Print and shaded views of the part. All mm, measured from the part's lowest x, y and z. A direction names the side the tool comes from. Coordinates: 2 decimals unless noted, no trailing zeros. Order: outer loops, then holes, each group sorted by start corner. A loop starts at its lowest first (then second) coordinate and runs counter-clockwise, first axis right, second up. Notation, with made-up numbers: (-26.75, -39.5) -> (28.25, -39.5) arc R25 cw to (28.25, -18.5) -> close; hole circle Ø10 at (73, -28.5). An arc over 180 degrees is marked (long way). Write item = value, one per line. Start each with the question number.
Q1. Cut at D-D, the plane y = 13.5. List the corners of the cut face in (x, z), plus the area to 3 significant figures.
Q2. 3-axis set-ups, long thin cutter, end or side, ignore diameter. For the marked faces 4, 5, 6, 7 and 8: which of +Z, -Z, +X, -X, +Y, -Y reach the whole face in a straight line?
Q3. Flat gauge pins, fed straight in: pin 1 (6.5 mm diameter, centred on x = 12.5, y = 5.5, fed in from -Z); pin 2 (4 mm diameter, centred on x = 14.5, z = 17.5, fed in from +Y); pin 3 (2 mm diameter, centred on x = 25.5, z = 36, fed in from -Y); pin 4 (4 mm diameter, centred on y = 12.5, z = 28, fed in from -X). Where does each tip first touch, or does it go through?
Q4. Cut at C-C, the plane z = 38. List the corners of the cut face in (x, y) (3 decimals).
Q5. Cut at A-A, the plane y = 24. List the corners of the cut face in (x, z).
Q6. Mould opens along X. For the marked faces 1, 2 and 3 say: +X half, -X half, draft (parallel to the pull), parting line (faces both ways), or undercut.
Q7. Cut at B-B, the plane x = 44. List the corners of the cut face in (y, z).
Q8. Wall check: line 1 (X direction, y = 31.5, z = 35.5); line 2 (Z direction, x = 28, y = 36.5); line 3 (Z direction, x = 61.5, y = 14). Give the ranges that are in metal, low to high. Write a range as from..to.
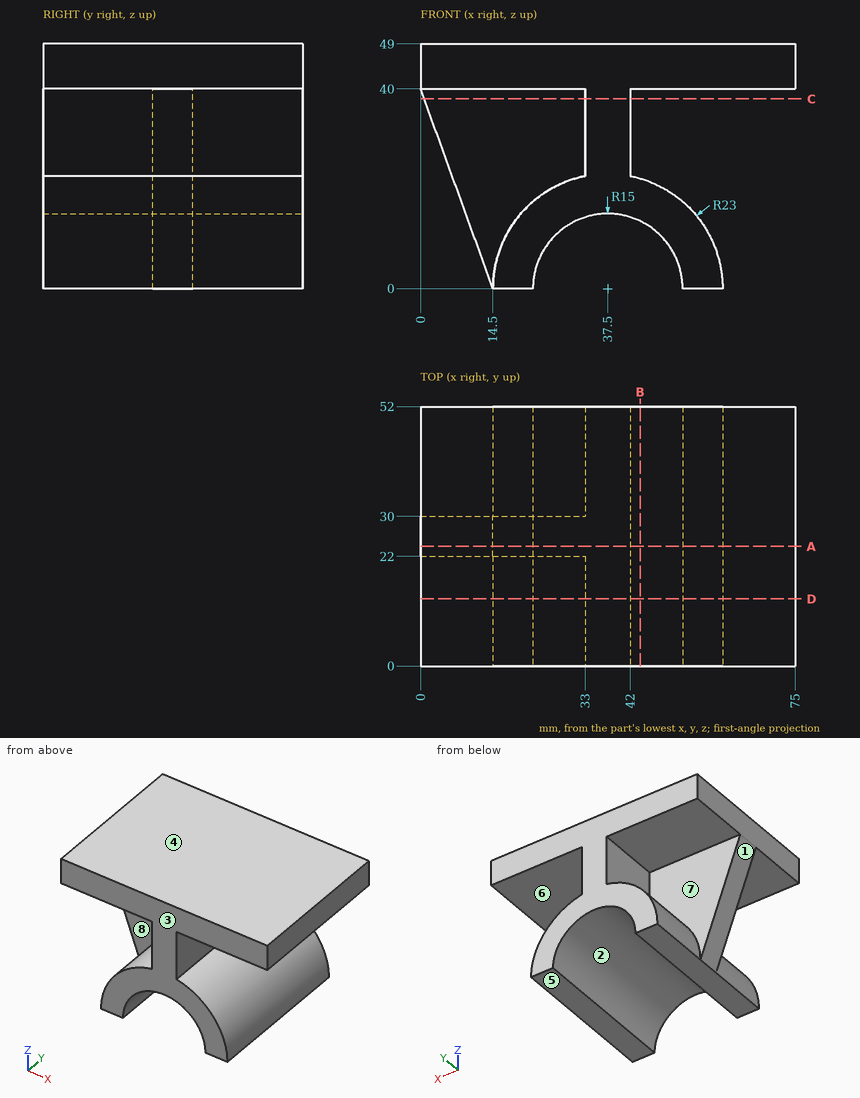
Here are the results:
q1.outline = (0, 40) -> (33, 40) -> (33, 22.56) arc R23 ccw to (14.5, 0) -> (22.5, 0) arc R15 cw to (52.5, 0) -> (60.5, 0) arc R23 ccw to (42, 22.56) -> (42, 40) -> (75, 40) -> (75, 49) -> (0, 49) -> close
q1.area = 1,310 mm²
q2.face_4 = +Z, +X, -X, +Y, -Y
q2.face_5 = -Z, +X, -X, +Y, -Y
q2.face_6 = +X, +Y, -Y
q2.face_7 = -X, +Y
q2.face_8 = -X, -Y
q3.pin_1 = 0
q3.pin_2 = 30
q3.pin_3 = 22
q3.pin_4 = 33
q4.outline = (0.725, 22) -> (33, 22) -> (33, 0) -> (42, 0) -> (42, 52) -> (33, 52) -> (33, 30) -> (0.725, 30) -> close
q5.outline = (0, 40) -> (14.5, 0) -> (22.5, 0) arc R15 cw to (52.5, 0) -> (60.5, 0) arc R23 ccw to (42, 22.56) -> (42, 40) -> (75, 40) -> (75, 49) -> (0, 49) -> close
q6.face_1 = -X half
q6.face_2 = undercut
q6.face_3 = draft
q7.outline = (0, 13.52) -> (52, 13.52) -> (52, 22.06) -> (0, 22.06) -> close; (0, 40) -> (52, 40) -> (52, 49) -> (0, 49) -> close
q8.line_1 = 33..42
q8.line_2 = 11.61..20.95, 40..49
q8.line_3 = 40..49
